The listing builds one solid part. Answer for the finished solid, in the listing's coordinates (mm). Face numbers are marked on the shaded views. A direction names the side the tool comes from. Give positions to 0.01 mm unless a question says otherwise; leave off trailing zeros. Order: outer loops, then holes, each group sorted by start corner. A loop starts at its lowest first (then second) coordinate and runs counter-clockwise, first axis right, second up.
```python
from build123d import *

# Parameters (mm, degrees)
PAD_DEPTH       = 15
SKETCH001_R     = 2.5
POCKET_DEPTH    = 6
PAD001_DEPTH    = 69
POCKET001_DEPTH = 0.001
POCKET002_DEPTH = 126.205435
SKETCH004_R     = 2.52796
SKETCH004_R_2   = 2.538571
POCKET003_DEPTH = 6


with BuildPart() as part:
    # Sketch → Pad (new body)
    with BuildSketch(Plane.YZ):
        Polygon((-126.204435, 0), (0, 0), (0, 5), (-7.071068, 12.071068), (-11.101576, 8.040559), (-72.619866, 69.558849), (-68.589358, 73.589358), (-90.509668, 95.509668), (-102.756291, 95.509668), (-126.204435, 8), align=None)
        with BuildLine():
            Line((-93.961967, 79.587241), (-27.868512, 13.493786))
            ThreePointArc((-30.144113, 8), (-27.170897, 9.986639), (-27.868512, 13.493786))
            Line((-30.144113, 8), (-112.060173, 8))
            ThreePointArc((-116.405015, 13.662309), (-115.628765, 9.759835), (-112.060173, 8))
            Line((-116.405015, 13.662309), (-99.110102, 78.207802))
            ThreePointArc((-93.961967, 79.587241), (-96.934244, 80.38366), (-99.110102, 78.207802))
        make_face(mode=Mode.SUBTRACT)
    extrude(amount=PAD_DEPTH)

    # Sketch001 (on Face8 of Pad) → Pocket (cut)
    with BuildSketch(Plane(origin=(0, 2.5, 2.5), x_dir=(0, -0.707107, 0.707107), z_dir=(0, 0.707107, 0.707107))):
        with Locations((8.535534, 7.61996)):
            Circle(SKETCH001_R)
        with Locations((124.535534, 7.619247)):
            Circle(SKETCH001_R)
    extrude(amount=-POCKET_DEPTH, mode=Mode.SUBTRACT)

    # Sketch002 (on Face5 of Pocket) → Pad001 (join)
    with BuildSketch(Plane.YZ.offset(15)):
        Polygon((-105.598321, 84.903066), (-79.903066, 84.903066), (-90.509668, 95.509668), (-102.756291, 95.509668), align=None)
    extrude(amount=PAD001_DEPTH)

    # Sketch003 → Pocket001 (cut, through all)
    with BuildSketch(Plane.XZ):
        Polygon((23, 95.509668), (29, 89.509668), (41, 89.509668), (47, 95.509668), align=None)
        Polygon((50, 95.509668), (74, 95.509668), (68, 89.509668), (56, 89.509668), align=None)
    extrude(amount=-POCKET001_DEPTH, mode=Mode.SUBTRACT)

    # Sketch003 → Pocket002 (cut, through all)
    with BuildSketch(Plane.XZ):
        Polygon((23, 95.509668), (29, 89.509668), (41, 89.509668), (47, 95.509668), align=None)
        Polygon((50, 95.509668), (74, 95.509668), (68, 89.509668), (56, 89.509668), align=None)
    extrude(amount=POCKET002_DEPTH, mode=Mode.SUBTRACT)

    # Sketch004 (on Face21 of Pocket002) → Pocket003 (cut)
    with BuildSketch(Plane(origin=(0, 0, 95.509668), x_dir=(0, -1, 0), z_dir=(0, 0, 1))):
        with Locations((99.509668, 19.5)):
            Circle(SKETCH004_R)
        with Locations((99.509668, 77.5)):
            Circle(SKETCH004_R_2)
    extrude(amount=-POCKET003_DEPTH, mode=Mode.SUBTRACT)


solid = part.part
```
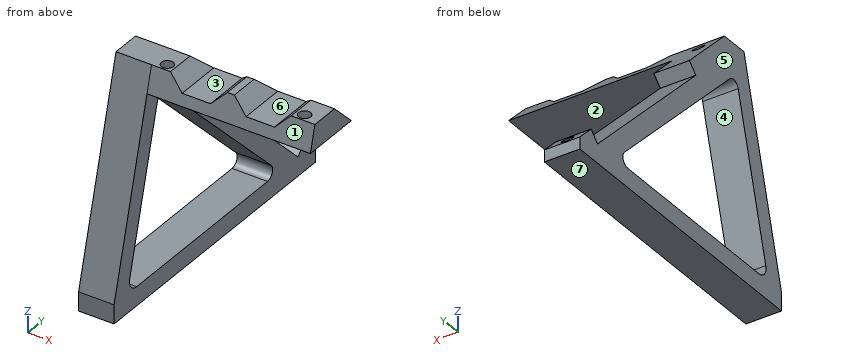
1) Find section A-A (y = -55). Write down the section's boundary in (x, z), then the cut area to 3 significant figures.
Geometry says:
outline: (0, 0) - (15, 0) - (15, 8) - (0, 8) - close; (0, 40.63) - (15, 40.63) - (15, 51.94) - (0, 51.94) - close
area: 290 mm2
2) Find section B-B (z = 40). Write down the section's boundary in (x, y), then the cut area to 3 significant figures.
Geometry says:
outline: (0, -117.63) - (15, -117.63) - (15, -109.35) - (0, -109.35) - close; (0, -54.37) - (15, -54.37) - (15, -43.06) - (0, -43.06) - close
area: 294 mm2
3) A tool of negligible diameter and unlimited length cuts with its end or side. For the marked faces 1, 2, 3 and 4, from which of +Z, -Z, +X, -X, +Y, -Y can it reach the whole face along a straight path? Write none if from no direction.
Geometry says:
face 1: +Z, +X, -X, -Y
face 2: -Z, +X, +Y, -Y
face 3: +Z, +Y, -Y
face 4: +X, -X
4) Given P1, Ø4, axis at x = 78, y = -99.5, coming from the +Z side; P2, Ø4, axis at x = 77.5, y = -99.51, coming from the -Z side; P3, Ø7.5, axis at x = 8, y = -77, coming from the +Z side, each flat-ended and moving along its own axis, determine where each tip first touches the part or whether it passes through.
Geometry says:
P1: stops at z = 89.51
P2: stops at z = 84.9
P3: stops at z = 85.75
5) Find section C-C (x = 77.5). Write down the section's boundary in (y, z), then the cut area to 3 significant figures.
Geometry says:
outline: (-105.6, 84.9) - (-79.9, 84.9) - (-90.51, 95.51) - (-96.97, 95.51) - (-96.97, 89.51) - (-102.05, 89.51) - (-102.05, 95.51) - (-102.76, 95.51) - close
area: 171 mm2
6) Find section D-D (x = 19.5). Write down the section's boundary in (y, z), then the cut area to 3 significant figures.
Geometry says:
outline: (-105.6, 84.9) - (-79.9, 84.9) - (-90.51, 95.51) - (-96.98, 95.51) - (-96.98, 89.51) - (-102.04, 89.51) - (-102.04, 95.51) - (-102.76, 95.51) - close
area: 171 mm2
7) Straight lines are drawn through the part: probe 1 along Z at (x, y) = (32, -98); probe 2 along Z at (x, y) = (8.5, -8); probe 3 along Z at (x, y) = (14.5, -61.5). For each, find the intervals that lie inside material, in ascending order.
Geometry says:
probe 1: z = 84.9 to 89.51
probe 2: z = 0 to 4.51, 7.38 to 11.14
probe 3: z = 0 to 8, 47.13 to 58.44
8) For a pull along X with two mould halves and no side action, classify the marked faces 5, 6 and 7 as +X half, -X half, draft (parallel to the pull), parting line (faces both ways), or undercut.
Geometry says:
face 5: -X half
face 6: undercut
face 7: draft
